Geometry: final body of the model. Coordinates: model frame, mm. Face numbers are marked on the shaded views. A direction names the side the tool comes from. Give positions to 0.01 mm unless a question says otherwise; leave off trailing zeros. Loops run counter-clockwise (first coordinate to the right, second up) from the corner with the lowest first, then second, coordinate; pieces in that order, holes last. Notation, with made-up numbers: (53, -16.5) - (98, -16.5) arc R17 cw to (98, -7.5) - close; hole circle Ø7 at (49, 15.5). An arc over 180 degrees is marked (long way). Use one line per item in the form item = value.
```python
from build123d import *

# Parameters (mm, degrees)
F0_W     = 107.95
F0_H     = 171.45
F0_W_2   = 88.9
F0_H_2   = 44.45
F1_DEPTH = 139.7
F2_W     = 107.95
F2_H     = 171.45
F3_DEPTH = 2.54
F5_DEPTH = 6.35


with BuildPart() as f1:
    # F0 (on Front) → F1 (new body)
    with BuildSketch(Plane.XZ):
        with Locations((-54.33191, 13.475312)):
            Rectangle(F0_W, F0_H)
        with Locations((-54.33191, -40.499688)):
            Rectangle(F0_W_2, F0_H_2, mode=Mode.SUBTRACT)
        with Locations((-54.33191, 67.450312)):
            Rectangle(F0_W_2, F0_H_2, mode=Mode.SUBTRACT)
        with Locations((-54.33191, 13.475312)):
            Rectangle(F0_W_2, F0_H_2, mode=Mode.SUBTRACT)
    extrude(amount=F1_DEPTH)

    # F2 (on face) → F3 (join)
    with BuildSketch(Plane(origin=(0, 0, 0), x_dir=(-1, 0, 0), z_dir=(0, 1, 0))):
        with Locations((54.33191, 13.475312)):
            Rectangle(F2_W, F2_H)
    extrude(amount=F3_DEPTH)

    # F4 (on face) → F5 (join)
    with BuildSketch(Plane(origin=(0, 2.54, 0), x_dir=(-1, 0, 0), z_dir=(0, 1, 0))):
        Polygon((121.00691, 111.900312), (0.35691, 111.900312), (-12.34309, 111.900312), (-12.34309, 99.200312), (-12.34309, -84.949688), (108.30691, -84.949688), (121.00691, -84.949688), (121.00691, -72.249688), align=None)
    extrude(amount=F5_DEPTH)


solid = f1.part
```
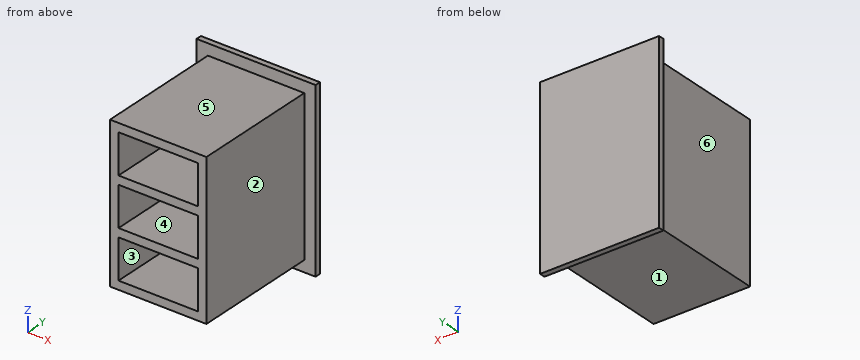
(1) Cut plane A-A (y = -63). Return the cut outline in (x, z).
Solution:
outline = (-108.31, -72.25) - (-0.36, -72.25) - (-0.36, 99.2) - (-108.31, 99.2) - close; hole (-98.78, -62.72) - (-9.88, -62.72) - (-9.88, -18.27) - (-98.78, -18.27) - close; hole (-98.78, -8.75) - (-9.88, -8.75) - (-9.88, 35.7) - (-98.78, 35.7) - close; hole (-98.78, 45.23) - (-9.88, 45.23) - (-9.88, 89.68) - (-98.78, 89.68) - close
(2) Cut plane C-C (x = -15). Return the cut outline in (y, z), plus the area to 3 significant figures.
Solution:
outline = (-139.7, -72.25) - (2.54, -72.25) - (2.54, -84.95) - (8.89, -84.95) - (8.89, 111.9) - (2.54, 111.9) - (2.54, 99.2) - (-139.7, 99.2) - (-139.7, 89.68) - (0, 89.68) - (0, 45.23) - (-139.7, 45.23) - (-139.7, 35.7) - (0, 35.7) - (0, -8.75) - (-139.7, -8.75) - (-139.7, -18.27) - (0, -18.27) - (0, -62.72) - (-139.7, -62.72) - close
area = 7,010 mm2
(3) Access query for the marked faces 1, 2 and 3. Directions: +Z, -Z, +X, -X, +Y, -Y. A direction counts if a zero-diameter tool reaches every point of the face in a straight line with its end or side. Return the directions, or none.
Solution:
face_1 = -Z, +X, -X, -Y
face_2 = +Z, -Z, +X, -Y
face_3 = -Y
(4) Material intervals for L1, parallel to Z at x = -61, y = -46; L2, parallel to X at y = -41, z = 82; L3, parallel to Y at x = -12, z = 71, sorted ascending. Write a range as from..to.
Solution:
L1 = -72.25..-62.72, -18.27..-8.75, 35.7..45.23, 89.68..99.2
L2 = -108.31..-98.78, -9.88..-0.36
L3 = 0..8.89
(5) Cut plane D-D (z = 39). Return the cut outline in (x, y), plus the area to 3 significant figures.
Solution:
outline = (-121.01, 2.54) - (-108.31, 2.54) - (-108.31, -139.7) - (-0.36, -139.7) - (-0.36, 2.54) - (12.34, 2.54) - (12.34, 8.89) - (-121.01, 8.89) - close
area = 16,200 mm2
(6) Pin query (flat end, axial travel): P1, Ø4, axis at x = -91, z = 20.5, coming from the -Y side; P2, Ø22, axis at y = -66, z = -38, coming from the -X side; P3, Ø13.5, axis at y = -71.5, z = -49.5, coming from the +X side. Return the tip coordinate at first contact, or that it passes through.
Solution:
P1 = 0
P2 = -108.31
P3 = -0.36
(7) Pull-direction query (Z, two-part tool) for the marked faces 4, 5 and 6; classes: released by +Z, released by -Z, zero draft, split by the parting line, or undercut.
Solution:
face_4 = undercut
face_5 = released by +Z
face_6 = zero draft
(8) Cut plane B-B (z = 69.5). Return the cut outline in (x, y), plus the area to 3 significant figures.
Solution:
outline = (-121.01, 2.54) - (-108.31, 2.54) - (-108.31, -139.7) - (-98.78, -139.7) - (-98.78, 0) - (-9.88, 0) - (-9.88, -139.7) - (-0.36, -139.7) - (-0.36, 2.54) - (12.34, 2.54) - (12.34, 8.89) - (-121.01, 8.89) - close
area = 3,780 mm2
